```python
from build123d import *

# Parameters (mm, degrees)
SKETCH1_R           = 1.5
BOSS_EXTRUDE1_DEPTH = 3


with BuildPart() as part:
    # Sketch1 → Boss-Extrude1 (new body)
    with BuildSketch(Plane(origin=(0, 0, 0), x_dir=(1, 0, 0), z_dir=(0, 1, 0))):
        with BuildLine():
            Line((-50, -10), (50, -10))
            ThreePointArc((50, -10), (57.071067812, -7.071067812), (60, 0))
            Line((60, 0), (60, 45))
            ThreePointArc((60, 45), (57.071067812, 52.071067812), (50, 55))
            Line((50, 55), (-50, 55))
            ThreePointArc((-50, 55), (-57.071067812, 52.071067812), (-60, 45))
            Line((-60, 45), (-60, 0))
            ThreePointArc((-60, 0), (-57.071067812, -7.071067812), (-50, -10))
        make_face()
        Circle(SKETCH1_R, mode=Mode.SUBTRACT)
        with Locations((0, 38)):
            Circle(SKETCH1_R, mode=Mode.SUBTRACT)
    extrude(amount=BOSS_EXTRUDE1_DEPTH)


solid = part.part
```
CAD build for the part. Positions are in the model's coordinates, mm. Give positions to 0.01 mm unless a question says otherwise; leave off trailing zeros. Order: outer loops, then holes, each group sorted by start corner. A loop starts at its lowest first (then second) coordinate and runs counter-clockwise, first axis right, second up.
(1) Flat gauge pins, fed straight in: pin 1 (1.8 mm diameter, centred on x = 0, z = -38, fed in from +Y); pin 2 (4 mm diameter, centred on x = -44.5, z = -28.5, fed in from -Y). Where does each tip first touch, or does it go through?
(2) Mould opens along X. For faces 1 (the cylindrical face through (57.15, 1.48, -51.99)), 2 (the flat face through (-1, 3, -23)), 3 (the cylindrical face through (-0.325, 1.479, -36.536)) say: released by +X, released by -X, zero draft, split by the parting line, or undercut.
(3) Drill centre lines: L1, parallel to Z at x = 0, y = 2.3; L2, parallel to Z at x = 0.5, y = 1.5; L3, parallel to X at y = 1.9, z = -38. Where is each one in solid material? Low to high.
(4) Saw through at A-A, the plane x = 0. Give the cut face in (y, z), then the cut area to 3 significant figures.
(5) Saw through at B-B, the plane z = -38. Give the cut face in (x, y), then the cut area to 3 significant figures.
Results found:
1. pin 1: passes through
1. pin 2: stops at y = 0
2. face 1: released by +X
2. face 2: zero draft
2. face 3: undercut
3. L1: z = -55 to -39.5, -36.5 to -1.5, 1.5 to 10
3. L2: z = -55 to -39.41, -36.59 to -1.41, 1.41 to 10
3. L3: x = -60 to -1.5, 1.5 to 60
4. outline: (0, -55) - (3, -55) - (3, -39.5) - (0, -39.5) - close; (0, -36.5) - (3, -36.5) - (3, -1.5) - (0, -1.5) - close; (0, 1.5) - (3, 1.5) - (3, 10) - (0, 10) - close
4. area: 177 mm2
5. outline: (-60, 0) - (-1.5, 0) - (-1.5, 3) - (-60, 3) - close; (1.5, 0) - (60, 0) - (60, 3) - (1.5, 3) - close
5. area: 351 mm2
